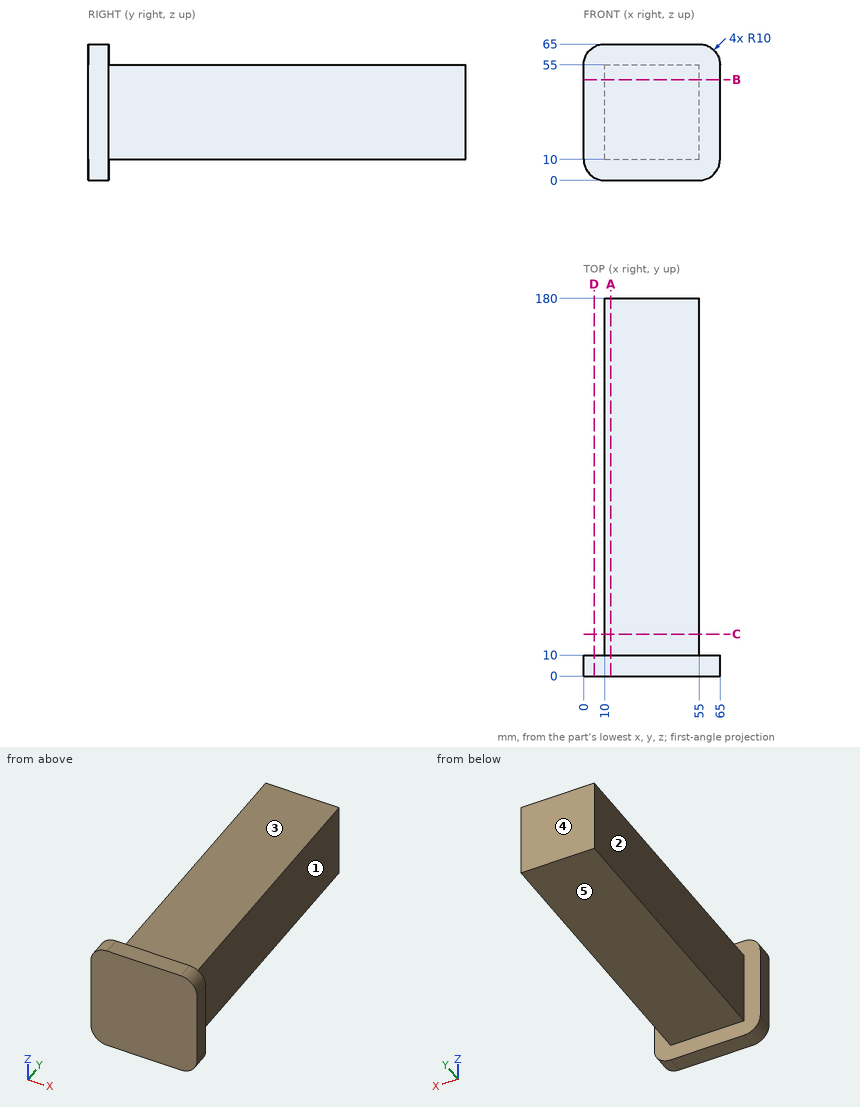
Answer from the drawing. Dimensions are ordinates in mm from the lowest x, y and z of the part. A direction names the side the tool comes from. Give positions to 0.01 mm unless a question says otherwise; leave off trailing zeros. Order: outer loops, then holes, each group sorted by start corner. A loop starts at its lowest first (then second) coordinate and runs counter-clockwise, first axis right, second up. Notation, with made-up numbers: (54.25, 66) - (102.25, 66) arc R31 cw to (102.25, 90) - close; hole circle Ø7 at (58.5, 44.25). An arc over 180 degrees is marked (long way). Use one line per item in the form item = value.
1) The mould has two halves that part along X. Classify the marked faces 1, 2 and 3: released by +X, released by -X, zero draft, split by the parting line, or undercut.
Verdict:
face_1 = released by +X
face_2 = released by -X
face_3 = zero draft
2) For the marked faces 4 and 5, determine the directions among +Z, -Z, +X, -X, +Y, -Y from which every point of the face is accessible in a straight line to the end or side of a thin tool.
Verdict:
face_4 = +Z, -Z, +X, -X, +Y
face_5 = -Z, +X, -X, +Y
3) Find section B-B on z = 48. Determine the outline of the cut face in (x, y).
Verdict:
outline = (0, 0) - (65, 0) - (65, 10) - (55, 10) - (55, 180) - (10, 180) - (10, 10) - (0, 10) - close
4) Consider probe 1 along X at (y, z) = (79, 28); probe 2 along Y at (x, z) = (45.5, 62.5). Determine where each line is inside the solid, lowest interval first. Write a range as [from, to].
Verdict:
probe_1 = [10, 55]
probe_2 = [0, 10]
5) Find section A-A on x = 13. Determine the outline of the cut face in (y, z), and give its area (3 significant figures).
Verdict:
outline = (0, 0) - (10, 0) - (10, 10) - (180, 10) - (180, 55) - (10, 55) - (10, 65) - (0, 65) - close
area = 8,300 mm^2
6) Find section D-D on x = 5. Determine the outline of the cut face in (y, z).
Verdict:
outline = (0, 1.34) - (10, 1.34) - (10, 63.66) - (0, 63.66) - close
7) Find section C-C on y = 20. Determine the outline of the cut face in (x, z).
Verdict:
outline = (10, 10) - (55, 10) - (55, 55) - (10, 55) - close
8) Each of these flat-tipped pins is pushed along its axis until it touches: pin 1 (5 mm diameter, centred on y = 56.5, z = 17.5, fed in from -X); pin 2 (13.5 mm diameter, centred on y = 89.5, z = 26, fed in from +X); pin 3 (22.5 mm diameter, centred on x = 30, y = 68, fed in from -Z). Where does it stop, or does it pass through?
Verdict:
pin_1 = 10
pin_2 = 55
pin_3 = 10
